Read the model definition and answer for the solid it produces. Units are mm, in the model's axes. A direction names the side the tool comes from. Give positions to 0.01 mm unless a question says otherwise; leave off trailing zeros. Write each loop counter-clockwise with the first axis right and the second up, starting at its lowest first coordinate (ties: lowest second). Pieces come first, ordered by that corner, then holes. Notation, with made-up numbers: (-8, 89) -> (25, 89) arc R33 cw to (25, 123) -> close; hole circle Ø11 at (17.25, 47.25). An arc over 180 degrees is marked (long way). Write item = value, one per line.
Autodesk Inventor part; units mm, degrees
ref_plane "YZ Plane" through (0, 0, 0) normal (1, 0, 0) x (0, 1, 0)
ref_plane "XZ Plane" through (0, 0, 0) normal (0, 1, 0) x (-1, 0, 0)
ref_plane "XY Plane" through (0, 0, 0) normal (0, 0, 1) x (1, 0, 0)
sketch "Sketch1" plane through (0, 0, 0) normal (0, 0, 1) x (1, 0, 0)
  line L0 (-20, 10) -> (20, 10)
  line L1 (20, 10) -> (20, -10)
  line L2 (20, -10) -> (-20, -10)
  line L3 (-20, -10) -> (-20, 10)
  line L4 (-20, 10) -> (20, -10) construction
  line L5 (20, 10) -> (-20, -10) construction
  line L6 (-27.5, 16) -> (27.5, 16)
  line L7 (27.5, 16) -> (27.5, -16)
  line L8 (27.5, -16) -> (-27.5, -16)
  line L9 (-27.5, -16) -> (-27.5, 16)
  line L10 (-27.5, 16) -> (27.5, -16) construction
  line L11 (27.5, 16) -> (-27.5, -16) construction
  line L12 (0, 0) -> (0, 16) construction
  circle A0 centre (-24, 0) radius 2.25
  circle A1 centre (24, 0) radius 2.25
  dimension "d0" = 40
  dimension "d1" = 20
  dimension "d2" = 32
  dimension "d3" = 55
  dimension "d4" = 4.5
  dimension "d5" = 24
extrude "Extrusion1" add sketch "Sketch1" along normal blind 6
chamfer "Chamfer1" distance 4.5 angle 45 4 edges at (27.5, 16, 3) (27.5, -16, 3) (-27.5, -16, 3) (-27.5, 16, 3)
sketch "Sketch3" plane through (0, 0, 6) normal (0, 0, 1) x (1, 0, 0)
  line L0 (-23, -16) -> (23, -16)
  line L1 (0, -16) -> (-18, -16)
  line L2 (-18, -16) -> (-18, -36)
  line L3 (-18, -36) -> (0, -36)
  line L4 (0, -36) -> (0, -16)
  circle A0 centre (-13.5, -24) radius 1.25
  line L5 (-13.5, -24) -> (-13.5, -32) construction
  circle A1 centre (-13.5, -32) radius 1.25
  line L6 (23, -16) -> (-23, -16)
  line L7 (18, -16) -> (18, -36)
  line L8 (18, -36) -> (0, -36)
  circle A2 centre (13.5, -24) radius 1.25
  circle A3 centre (13.5, -32) radius 1.25
  line L9 (-27.5, 11.5) -> (-27.5, -11.5)
  point P0 (0, 0)
  dimension "d17" = 18
  dimension "d18" = 20
  dimension "d19" = 2.5
  dimension "d20" = 2.5
  dimension "d21" = 8
  dimension "d22" = 16
  dimension "d26" = 13.5
extrude "Extrusion3" add sketch "Sketch3" against normal blind 6
chamfer "Chamfer2" distance 4.5 angle 45 2 edges at (18, -36, 3) (-18, -36, 3)
sketch "Sketch6" plane through (0, 0, 0) normal (0, 0, -1) x (-1, 0, 0)
  line L0 (20, 10) -> (-20, 10)
  line L1 (-23, 16) -> (23, 16)
  line L2 (-20, 10) -> (20, 10)
  line L3 (20, 10) -> (20, 16)
  line L4 (20, 16) -> (-20, 16)
  line L5 (-20, 16) -> (-20, 10)
  point P0 (0, 0)
  dimension "d30" = 40
extrude "Extrusion4" add sketch "Sketch6" along normal blind 30
chamfer "Chamfer3" distance 4.5 angle 45 3 edges at (-20, 16, -15) (20, 16, -15) (0, 16, -30)
sketch "Sketch2" plane through (-23, 16, 0) normal (0, 1, 0) x (1, 0, 0)
  line L0 (50.5, -6) -> (50.5, 0)
  line L1 (50.5, -3) -> (-4.5, -3) construction
  line L2 (-4.5, 0) -> (-4.5, -6)
  line L3 (23, 0) -> (23, -6) construction
  line L4 (33, -3) -> (33, 2)
  circle A0 centre (33, 2) radius 2
  circle A1 centre (13, 2) radius 2
  circle A2 centre (33, 22) radius 2
  circle A3 centre (13, 22) radius 2
  dimension "d11" = 10
  dimension "d36" = 5
  dimension "d37" = 4
  dimension "d40" = 20
  dimension "d43" = 20
extrude "Extrusion2" cut sketch "Sketch2" against normal blind 10
properties part number "ServoCarrier"
(1) The part is cut by section D-D on z = 2. Determine the outline of the cut face in (x, y), plus the area to 3 significant figures.
Checks:
outline = (-27.5, -11.5) -> (-23, -16) -> (-18, -16) -> (-18, -31.5) -> (-13.5, -36) -> (13.5, -36) -> (18, -31.5) -> (18, -16) -> (23, -16) -> (27.5, -11.5) -> (27.5, 11.5) -> (23, 16) -> (-23, 16) -> (-27.5, 11.5) -> close; hole circle Ø4.5 at (-24, 0); hole (-20, -10) -> (20, -10) -> (20, 10) -> (-20, 10) -> close; hole circle Ø2.5 at (-13.5, -32); hole circle Ø2.5 at (-13.5, -24); hole circle Ø2.5 at (13.5, -32); hole circle Ø2.5 at (13.5, -24); hole circle Ø4.5 at (24, 0)
area = 1,570 mm²
(2) The part is cut by section C-C on x = 10. Determine the outline of the cut face in (y, z).
Checks:
outline = (-36, 0) -> (-10, 0) -> (-10, 6) -> (-36, 6) -> close; (10, -30) -> (11.5, -30) -> (16, -25.5) -> (16, -24) -> (10, -24) -> close; (10, -20) -> (16, -20) -> (16, -4) -> (10, -4) -> close; (10, 0) -> (16, 0) -> (16, 6) -> (10, 6) -> close
(3) The part is cut by section A-A on z = -22. Determine the outline of the cut face in (x, y).
Checks:
outline = (-20, 10) -> (-12, 10) -> (-12, 16) -> (-15.5, 16) -> (-20, 11.5) -> close; (-8, 10) -> (8, 10) -> (8, 16) -> (-8, 16) -> close; (12, 10) -> (20, 10) -> (20, 11.5) -> (15.5, 16) -> (12, 16) -> close
(4) Given P1, Ø10, axis at x = 6, y = 2, coming from the -Z side; P2, Ø4, axis at x = 10, z = -5.5, coming from the -Y side; P3, Ø6.5, axis at y = -20.5, z = 4.5, coming from the +X side; P4, Ø3, axis at x = -13.5, y = -32, coming from the -Z side, each flat-ended and moving along its own axis, determine where each tip first touches the part or whether it passes through.
Checks:
P1 = through
P2 = 10
P3 = 18
P4 = 0
(5) For a pull along X with two mould halves and no side action, classify faces 4 (the flat face through (0, -10, 3)), 5 (the flat face through (0, -36, 3)), 6 (the cylindrical face through (8.4, 13, -20.8)), 7 (the flat face through (-25, -14, 3)) as released by +X, released by -X, zero draft, split by the parting line, or undercut.
Checks:
face_4 = undercut
face_5 = zero draft
face_6 = undercut
face_7 = released by -X
(6) The part is cut by section B-B on x = -24. Determine the outline of the cut face in (y, z), plus the area to 3 significant figures.
Checks:
outline = (-15, 0) -> (-2.25, 0) -> (-2.25, 6) -> (-15, 6) -> close; (2.25, 0) -> (15, 0) -> (15, 6) -> (2.25, 6) -> close
area = 153 mm²
(7) A tool of negligible diameter and unlimited length cuts with its end or side. For faces 1 (the flat face through (20, 0, 3)), 2 (the flat face through (-20, -16, 3)), 3 (the flat face through (-27.5, 0, 3)), from which of +Z, -Z, +X, -X, +Y, -Y can it reach the whole face along a straight path? Write none if from no direction.
Checks:
face_1 = +Z, -Z
face_2 = +Z, -Z, -X, -Y
face_3 = +Z, -Z, -X, +Y, -Y
(8) Consider L1, parallel to Y at x = -13.5, z = 2.95; L2, parallel to Y at x = -6, z = 3.5; L3, parallel to X at y = 14, z = -22. Determine where each line is inside the solid, lowest interval first.
Checks:
L1 = -36 to -33.25, -30.75 to -25.25, -22.75 to -10, 10 to 16
L2 = -36 to -10, 10 to 16
L3 = -17.5 to -12, -8 to 8, 12 to 17.5
